Source: CAD feature listing. Evaluate the final solid. Frame: model axes, mm. Face numbers are marked on the shaded views. A direction names the side the tool comes from. Give positions to 0.01 mm unless a question says otherwise; leave off trailing zeros. Loops run counter-clockwise (first coordinate to the right, second up) from the corner with the lowest first, then second, coordinate; pieces in that order, holes last. Notation, with made-up numbers: M -39.5,29 L 19.5,29 A35 ccw 19.5,64 Z; hole C 21,50.25 d11. An arc over 180 degrees is marked long. Write item = value, one per line.
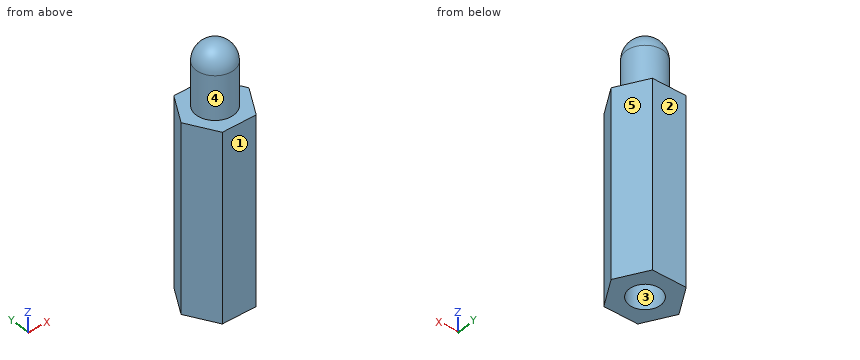
from build123d import *

# Parameters (mm, degrees)
EXTRUDE_1_DEPTH     = 15
SKETCH_2_R          = 1.5
EXTRUDE_2_DEPTH     = 5
FILLET_1_R          = 1.5
SKETCH_3_R          = 1.25
CUT_EXTRUDE_1_DEPTH = 10


with BuildPart() as part:
    # 草图1 → 凸台-拉伸1 (new body)
    with BuildSketch(Plane.XY):
        Polygon((2.690452254, 0), (1.345226127, 2.33), (-1.345226127, 2.33), (-2.690452254, 0), (-1.345226127, -2.33), (1.345226127, -2.33), align=None)
    extrude(amount=EXTRUDE_1_DEPTH)

    # 草图2 → 凸台-拉伸2 (add)
    with BuildSketch(Plane.XY.offset(15)):
        Circle(SKETCH_2_R)
    extrude(amount=EXTRUDE_2_DEPTH)

    # 圆角1
    fillet_1_edges = [part.edges().sort_by_distance(p)[0] for p in [
        (-1.5, 0, 20),
    ]]
    fillet(fillet_1_edges, radius=FILLET_1_R)

    # 草图3 → 切除-拉伸1 (cut)
    with BuildSketch(Plane(origin=(0, 0, 0), x_dir=(-1, 0, 0), z_dir=(0, 0, -1))):
        Circle(SKETCH_3_R)
    extrude(amount=-CUT_EXTRUDE_1_DEPTH, mode=Mode.SUBTRACT)


solid = part.part
1. Cut plane B-B, the plane x = 0. Return the cut outline in (y, z).
Derived:
outline = M -2.33,0 L -1.25,0 L -1.25,10 L 1.25,10 L 1.25,0 L 2.33,0 L 2.33,15 L 1.5,15 L 1.5,18.5 A1.5 ccw -1.5,18.5 L -1.5,15 L -2.33,15 Z
2. Material intervals for probe 1 along Y at (x, z) = (0, 7.75); probe 2 along Z at (x, y) = (-0.9, 1.3); probe 3 along Y at (x, z) = (-0.75, 3.75), sorted ascending. Write a range as from..to.
Derived:
probe_1 = -2.33..-1.25, 1.25..2.33
probe_2 = 0..15
probe_3 = -2.33..-1, 1..2.33
3. First-contact query: pin 1 Ø1 at (x, y) = (2, -1.5) entering from +Z; pin 2 Ø1.4 at (x, y) = (0.5, -0.5) entering from +Z; pin 3 Ø0.8 at (x, y) = (-0.5, 0) entering from -Z. Flat tips, straight axial feed; report the tip coordinate or a pass-through.
Derived:
pin_1 = 15
pin_2 = 20
pin_3 = 10
4. Cut plane C-C, the plane y = -0.6. Return the cut outline in (x, z), then the cut area to 3 significant figures.
Derived:
outline = M -2.34,0 L -1.1,0 L -1.1,10 L 1.1,10 L 1.1,0 L 2.34,0 L 2.34,15 L 1.37,15 L 1.37,18.5 A1.37 ccw -1.37,18.5 L -1.37,15 L -2.34,15 Z
area = 61.0 mm²
5. Reachability of the marked faces 4 and 5 from +Z, -Z, +X, -X, +Y, -Y: full face, straight path, thin tool, end or side. Return the list, or none.
Derived:
face_4 = +Z
face_5 = +Z, -Z, +X, +Y
6. Cut plane A-A, the plane z = 3.5. Return the cut outline in (x, y).
Derived:
outline = M -2.69,0 L -1.35,-2.33 L 1.35,-2.33 L 2.69,0 L 1.35,2.33 L -1.35,2.33 Z; hole C 0,0 d2.5
7. Cut plane D-D, the plane z = 14.5. Return the cut outline in (x, y), then the cut area to 3 significant figures.
Derived:
outline = M -2.69,0 L -1.35,-2.33 L 1.35,-2.33 L 2.69,0 L 1.35,2.33 L -1.35,2.33 Z
area = 18.8 mm²
8. Pull-direction query (Y, two-part tool) for the marked faces 1, 2 and 3; classes: +Y half, -Y half, draft (parallel to the pull), parting line (faces both ways), or undercut.
Derived:
face_1 = -Y half
face_2 = +Y half
face_3 = undercut
